Verification items for this drawing (mm, ordinates from the low corner). A direction names the side the tool comes from. Round coordinates to 2 decimals unless told otherwise and drop trailing zeros. Write each loop counter-clockwise with the first axis right and the second up, starting at its lowest first coordinate (ties: lowest second). Pieces come first, ordered by that corner, then holes.
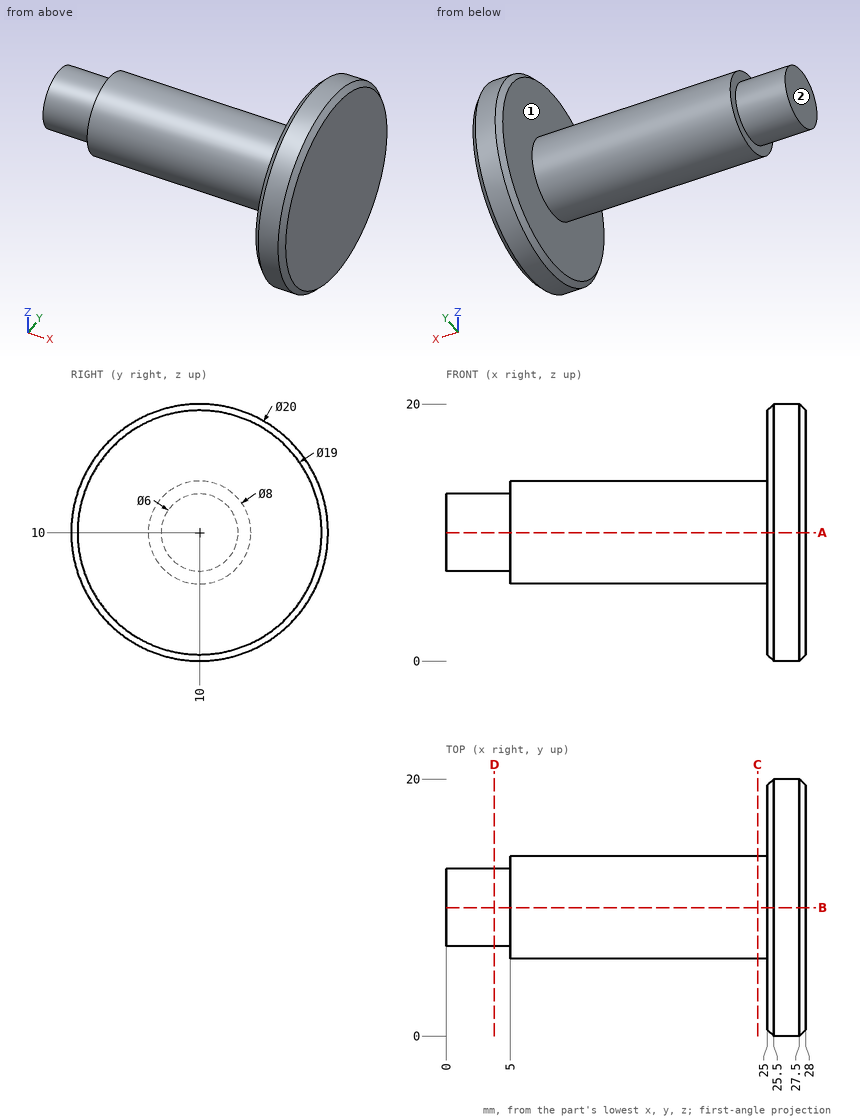
1. Section check D-D (x = 3.75). Record the cut outline in (y, z).
2. Scan lines: line 1 along X through (y, z) = (5.75, 13.5); line 2 along Z through (x, y) = (7.25, 10); line 3 along Y through (x, z) = (13, 6.5). Record each from-to range of solid material in increasing order.
3. Depth check by flat-ended pin: pin 1 Ø3 at (y, z) = (3, 2) entering from -X; pin 2 Ø3 at (x, z) = (5, 8) entering from +Y; pin 3 Ø3 at (x, z) = (8, 12) entering from -Y. Enter the tip coordinate at first touch or a pass-through.
4. Section check A-A (z = 10). Record the cut outline in (x, y).
5. Access from +Z, -Z, +X, -X, +Y, -Y to the whole of each face (thin tool, end or side, straight path). Record for the marked faces 1 and 2.
6. Section check C-C (x = 24.25). Record the cut outline in (y, z).
Results below:
1. outline: circle Ø6 at (10, 10)
2. line 1: x = 25 to 28
2. line 2: z = 6 to 14
2. line 3: y = 8.06 to 11.94
3. pin 1: stops at x = 25
3. pin 2: stops at y = 13.97
3. pin 3: stops at y = 6.03
4. outline: (0, 7) - (5, 7) - (5, 6) - (25, 6) - (25, 0.5) - (25.5, 0) - (27.5, 0) - (28, 0.5) - (28, 19.5) - (27.5, 20) - (25.5, 20) - (25, 19.5) - (25, 14) - (5, 14) - (5, 13) - (0, 13) - close
5. face 1: -X
5. face 2: +Z, -Z, -X, +Y, -Y
6. outline: circle Ø8 at (10, 10)
